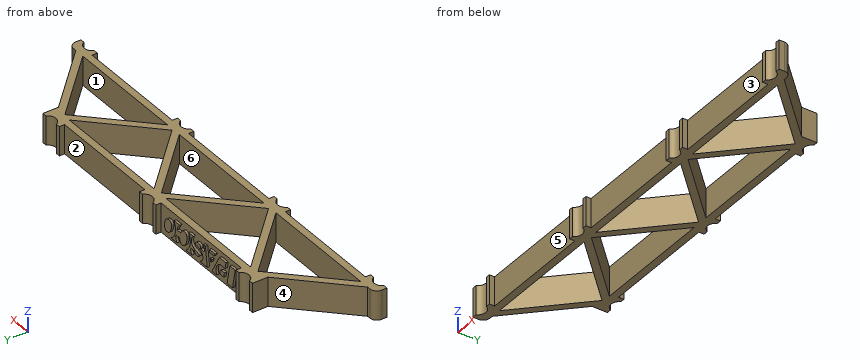
from build123d import *

# Parameters (mm, degrees)
BOSS_EXTRUDE1_DEPTH  = 3.175
BOSS_EXTRUDE2_DEPTH  = 3.175
BOSS_EXTRUDE3_START  = -3.175
BOSS_EXTRUDE3_DEPTH  = 6.35
FILLET1_R            = 1.524
FILLET1_OF_MIRROR1_R = 1.524
BOSS_EXTRUDE4_DEPTH  = 0.508


with BuildPart() as part:
    # Sketch1 → Boss-Extrude1 (new body, symmetric)
    with BuildSketch(Plane.XY):
        Polygon((-46.839630735, -15.762), (-30.315630735, 0.762), (0, 0.762), (30.315630735, 0.762), (46.839630735, -15.762), (15, -15.762), (-15, -15.762), align=None)
        Polygon((-43.160369265, -14.238), (-30, -1.077630735), (-16.839630735, -14.238), align=None, mode=Mode.SUBTRACT)
        Polygon((-28.160369265, -0.762), (-15, -13.922369265), (-1.839630735, -0.762), align=None, mode=Mode.SUBTRACT)
        Polygon((-13.160369265, -14.238), (0, -1.077630735), (13.160369265, -14.238), align=None, mode=Mode.SUBTRACT)
        Polygon((1.839630735, -0.762), (15, -13.922369265), (28.160369265, -0.762), align=None, mode=Mode.SUBTRACT)
        Polygon((16.839630735, -14.238), (30, -1.077630735), (43.160369265, -14.238), align=None, mode=Mode.SUBTRACT)
    extrude(amount=BOSS_EXTRUDE1_DEPTH, both=True)

    # Sketch2 → Boss-Extrude2 (add, symmetric)
    with BuildSketch(Plane.XY):
        with BuildLine():
            Line((-46.606437051, -16.905), (-47.54, -16.905))
            Line((-47.54, -16.905), (-47.54, -14.238))
            Line((-47.54, -14.238), (-42.46, -14.238))
            Line((-42.46, -14.238), (-42.46, -16.905))
            Line((-42.46, -16.905), (-43.393562949, -16.905))
            ThreePointArc((-43.393562949, -16.905), (-45, -15.889), (-46.606437051, -16.905))
        make_face()
        with BuildLine():
            Line((-27.46, 0.762), (-30.315630735, 0.762))
            Line((-30.315630735, 0.762), (-32.54, -1.462369265))
            Line((-32.54, -1.462369265), (-32.54, 0.762))
            Line((-32.54, 0.762), (-32.54, 1.905))
            Line((-32.54, 1.905), (-31.606437051, 1.905))
            ThreePointArc((-31.606437051, 1.905), (-30, 0.889), (-28.393562949, 1.905))
            Line((-28.393562949, 1.905), (-27.46, 1.905))
            Line((-27.46, 1.905), (-27.46, 0.762))
        make_face()
        with BuildLine():
            Line((-16.606437051, -16.905), (-17.54, -16.905))
            Line((-17.54, -16.905), (-17.54, -15.762))
            Line((-17.54, -15.762), (-12.46, -15.762))
            Line((-12.46, -15.762), (-12.46, -16.905))
            Line((-12.46, -16.905), (-13.393562949, -16.905))
            ThreePointArc((-13.393562949, -16.905), (-15, -15.889), (-16.606437051, -16.905))
        make_face()
    boss_extrude2 = extrude(amount=BOSS_EXTRUDE2_DEPTH, both=True)

    # Sketch3 → Boss-Extrude3 (add)
    with BuildSketch(Plane.XY.offset(BOSS_EXTRUDE3_START)):
        with BuildLine():
            Line((1.606437051, 1.905), (2.54, 1.905))
            Line((2.54, 1.905), (2.54, 0.762))
            Line((2.54, 0.762), (-2.54, 0.762))
            Line((-2.54, 0.762), (-2.54, 1.905))
            Line((-2.54, 1.905), (-1.606437051, 1.905))
            ThreePointArc((-1.606437051, 1.905), (0, 0.889), (1.606437051, 1.905))
        make_face()
    extrude(amount=BOSS_EXTRUDE3_DEPTH)

    # Fillet1
    fillet1_edges = [part.edges().sort_by_distance(p)[0] for p in [
        (-47.54, -14.238, 0),
    ]]
    fillet(fillet1_edges, radius=FILLET1_R)

    # Mirror1: Boss-Extrude2 across plane
    add(boss_extrude2.mirror(Plane(origin=(0, 0, 0), x_dir=(0, 0, 1), z_dir=(1, 0, 0))))

    # Fillet1 of Mirror1
    fillet1_of_mirror1_edges = [part.edges().sort_by_distance(p)[0] for p in [
        (47.54, -14.238, 0),
    ]]
    fillet(fillet1_of_mirror1_edges, radius=FILLET1_OF_MIRROR1_R)

    # Sketch4 → Boss-Extrude4 (add)
    with BuildSketch(Plane(origin=(30.341470111, 0.762, -10.998323426), x_dir=(-1, 0, 0), z_dir=(0, 1, 0))):
        Polygon((55.766638301, 8.903049935), (54.0821519, 8.903049935), (54.924395101, 13.184452869), (56.608881501, 13.184452869), align=None)
        with BuildLine():
            Line((49.373679321, 8.903049935), (51.695796166, 13.184452869))
            Line((51.695796166, 13.184452869), (53.731217234, 13.184452869))
            Line((53.731217234, 13.184452869), (53.455071922, 11.780714202))
            Line((53.455071922, 11.780714202), (52.044845481, 11.780714202))
            ThreePointArc((52.044845481, 11.780714202), (51.895660414, 11.763021636), (51.754751921, 11.710925494))
            ThreePointArc((51.754751921, 11.710925494), (50.74099205, 10.52746368), (50.853552966, 8.973236868))
            Line((50.853552966, 8.973236868), (50.888554794, 8.903049935))
            Line((50.888554794, 8.903049935), (49.373679321, 8.903049935))
        make_face()
        with BuildLine():
            Line((47.344206299, 13.184452869), (47.92473551, 8.903049935))
            Line((47.92473551, 8.903049935), (45.657455804, 8.903049935))
            Line((45.657455804, 8.903049935), (45.800093765, 8.973236868))
            ThreePointArc((45.800093765, 8.973236868), (46.559919921, 9.999679495), (46.16385217, 11.213784347))
            ThreePointArc((46.16385217, 11.213784347), (46.087708374, 11.278047887), (46.002485287, 11.329668676))
            ThreePointArc((46.002485287, 11.329668676), (45.241879319, 11.641820064), (44.44239948, 11.833632247))
            ThreePointArc((44.44239948, 11.833632247), (44.321830206, 11.897125178), (44.264573877, 12.020777977))
            ThreePointArc((44.264573877, 12.020777977), (44.273299822, 12.151811254), (44.326168164, 12.272022736))
            ThreePointArc((44.326168164, 12.272022736), (44.436687002, 12.409847066), (44.584321098, 12.50687352))
            ThreePointArc((44.584321098, 12.50687352), (45.07356558, 12.617554773), (45.566896159, 12.526805434))
            ThreePointArc((45.566896159, 12.526805434), (45.796502387, 12.340831934), (45.882880346, 12.05826511))
            Line((45.882880346, 12.05826511), (45.882880346, 11.780714202))
            Line((45.882880346, 11.780714202), (46.993271632, 11.780714202))
            ThreePointArc((46.993271632, 11.780714202), (47.00184458, 12.512372899), (46.712523898, 13.184452869))
            Line((46.712523898, 13.184452869), (47.344206299, 13.184452869))
        make_face()
        with BuildLine():
            Line((52.362572033, 10.727910202), (53.247962938, 10.727910202))
            Line((53.247962938, 10.727910202), (53.040853955, 9.675106202))
            Line((53.040853955, 9.675106202), (52.224130208, 9.675106202))
            ThreePointArc((52.224130208, 9.675106202), (51.949800938, 9.788737106), (51.836170033, 10.063066377))
            Line((51.836170033, 10.063066377), (51.836170033, 10.201508202))
            ThreePointArc((51.836170033, 10.201508202), (51.990349609, 10.573730626), (52.362572033, 10.727910202))
        make_face()
        Polygon((48.958505766, 10.596309702), (48.845492907, 11.429779536), (49.410557201, 11.429779536), align=None)
        Polygon((48.607571099, 13.184452869), (50.362244433, 13.184452869), (50.019637029, 12.552770469), (48.69322295, 12.552770469), align=None)
        with BuildLine():
            Line((43.093358174, 9.007864255), (43.203837606, 8.897384823))
            Line((43.203837606, 8.897384823), (41.238603472, 8.897384823))
            ThreePointArc((41.238603472, 8.897384823), (42.59037643, 10.850382179), (42.150373231, 13.184452869))
            Line((42.150373231, 13.184452869), (43.624298831, 13.184452869))
            ThreePointArc((43.624298831, 13.184452869), (42.976922737, 12.00046329), (43.609533036, 10.808518937))
            ThreePointArc((43.609533036, 10.808518937), (43.801404112, 10.703005905), (44.00849344, 10.63186155))
            Line((44.00849344, 10.63186155), (45.137184548, 10.349688773))
            ThreePointArc((45.137184548, 10.349688773), (45.325274084, 10.217067986), (45.375126192, 9.992388851))
            ThreePointArc((45.375126192, 9.992388851), (45.276758726, 9.771226443), (45.079326395, 9.631192719))
            ThreePointArc((45.079326395, 9.631192719), (44.392498989, 9.682709209), (43.976922089, 10.231964773))
            Line((43.976922089, 10.231964773), (42.853931155, 10.231964773))
            ThreePointArc((42.853931155, 10.231964773), (42.786913393, 9.583390951), (43.093358174, 9.007864255))
        make_face()
        with BuildLine():
            Line((38.57083963, 8.903049935), (36.605605496, 8.903049935))
            ThreePointArc((36.605605496, 8.903049935), (38.014670833, 10.833118693), (37.588222563, 13.184452869))
            Line((37.588222563, 13.184452869), (39.342895896, 13.184452869))
            ThreePointArc((39.342895896, 13.184452869), (38.831372076, 12.513225905), (38.57083963, 11.710527269))
            Line((38.57083963, 11.710527269), (39.693830563, 11.710527269))
            ThreePointArc((39.693830563, 11.710527269), (39.959617235, 12.233880985), (40.415270694, 12.603910164))
            ThreePointArc((40.415270694, 12.603910164), (41.166876497, 12.593701608), (41.591788981, 11.973649288))
            ThreePointArc((41.591788981, 11.973649288), (41.543037796, 10.949193829), (41.155213354, 9.999731945))
            ThreePointArc((41.155213354, 9.999731945), (40.782487914, 9.571566118), (40.251107207, 9.371854393))
            ThreePointArc((40.251107207, 9.371854393), (39.531077174, 9.674914925), (39.41308283, 10.447162469))
            Line((39.41308283, 10.447162469), (38.149718029, 10.447162469))
            ThreePointArc((38.149718029, 10.447162469), (38.201808334, 9.631886976), (38.57083963, 8.903049935))
        make_face()
        with BuildLine():
            Line((35.48104333, 9.602571887), (35.356873428, 9.602571887))
            ThreePointArc((35.356873428, 9.602571887), (34.923728887, 9.759646665), (34.691948891, 10.157848515))
            ThreePointArc((34.691948891, 10.157848515), (34.675735454, 10.986379145), (34.920455715, 11.778110082))
            ThreePointArc((34.920455715, 11.778110082), (35.261440878, 12.213116508), (35.747757566, 12.475790357))
            ThreePointArc((35.747757566, 12.475790357), (35.911443016, 12.505405638), (36.077655631, 12.511990293))
            ThreePointArc((36.077655631, 12.511990293), (36.647671195, 12.253324316), (36.864077445, 11.665962276))
            ThreePointArc((36.864077445, 11.665962276), (36.699639375, 10.801331502), (36.294750409, 10.019864179))
            ThreePointArc((36.294750409, 10.019864179), (35.938277424, 9.712977507), (35.48104333, 9.602571887))
        make_face()
    extrude(amount=BOSS_EXTRUDE4_DEPTH)


solid = part.part
Read the model definition and answer for the solid it produces. Units are mm, in the model's axes. Face numbers are marked on the shaded views. A direction names the side the tool comes from. Round coordinates to 2 decimals unless told otherwise and drop trailing zeros. Loops run counter-clockwise (first coordinate to the right, second up) from the corner with the lowest first, then second, coordinate; pieces in that order, holes last.
Q1. Section B-B on y = -6 is taken. Write down the section's boundary in (x, z) (3 decimals).
Q2. Consider probe 1 along Y at (x, z) = (6, -2.25); probe 2 along X at (y, z) = (-12.5, -0.75); probe 3 along X at (y, z) = (-11.5, 0.75). Determine where each line is inside the solid, lowest interval first.
Q3. Determine the mould class of the marked faces 4, 5 and 6 for opening direction Y: released by +Y, released by -Y, zero draft, split by the parting line, or undercut.
Q4. Section C-C on x = 4 is taken. Write down the section's boundary in (y, z) (3 decimals), and give its area (3 significant figures).
Q5. Section A-A on x = -39 is taken. Write down the section's boundary in (y, z) (3 decimals).
Q6. Each of these flat-tipped pins is pushed along its axis until it touches: pin 1 (2 mm diameter, centred on x = 3.5, y = -1, fed in from -Z) (3 decimals); pin 2 (2 mm diameter, centred on y = -2, z = 1, fed in from -X); pin 3 (2 mm diameter, centred on x = -10, z = 1, fed in from +Y); pin 4 (3.5 mm diameter, centred on y = 0, z = 0.5, fed in from +X). Where does it stop, or does it pass through?
Q7. Which of the six approach directions +Z, -Z, +X, -X, +Y, -Y give full straight-line access (tool end or side, diameter ignored) to the marked faces 1, 2 and 3?
Output:
1. outline: (-37.078, -3.175) - (-34.922, -3.175) - (-34.922, 3.175) - (-37.078, 3.175) - close; (-25.078, -3.175) - (-22.922, -3.175) - (-22.922, 3.175) - (-25.078, 3.175) - close; (-7.078, -3.175) - (-4.922, -3.175) - (-4.922, 3.175) - (-7.078, 3.175) - close; (4.922, -3.175) - (7.078, -3.175) - (7.078, 3.175) - (4.922, 3.175) - close; (22.922, -3.175) - (25.078, -3.175) - (25.078, 3.175) - (22.922, 3.175) - close; (34.922, -3.175) - (37.078, -3.175) - (37.078, 3.175) - (34.922, 3.175) - close
2. probe 1: y = -15.76 to -14.24, -7.08 to -4.92, -0.76 to 0.76
2. probe 2: x = -43.58 to -41.42, -18.58 to -16.42, -13.58 to -11.42, 11.42 to 13.58, 16.42 to 18.58, 41.42 to 43.58
2. probe 3: x = -42.58 to -40.42, -19.58 to -17.42, -12.58 to -10.42, 10.42 to 12.58, 17.42 to 19.58, 40.42 to 42.58
3. face 4: released by +Y
3. face 5: released by -Y
3. face 6: undercut
4. outline: (-15.762, -3.175) - (-14.238, -3.175) - (-14.238, 3.175) - (-15.762, 3.175) - close; (-5.078, -3.175) - (-2.922, -3.175) - (-2.922, 3.175) - (-5.078, 3.175) - close; (-0.762, -3.175) - (0.762, -3.175) - (0.762, 3.175) - (-0.762, 3.175) - close
4. area: 33.0 mm2
5. outline: (-15.762, -3.175) - (-14.238, -3.175) - (-14.238, 3.175) - (-15.762, 3.175) - close; (-10.078, -3.175) - (-7.922, -3.175) - (-7.922, 3.175) - (-10.078, 3.175) - close
6. pin 1: stops at z = -3.175
6. pin 2: stops at x = -34.08
6. pin 3: stops at y = 1.27
6. pin 4: stops at x = 32.83
7. face 1: +Z, -Z
7. face 2: +Z, -Z, +Y
7. face 3: +Z, -Z, -Y
